from build123d import *

# Parameters (mm, degrees)
SKETCH_1_W      = 15
SKETCH_1_H      = 10
EXTRUDE_1_DEPTH = 5
FILLET_1_R      = 1.2


with BuildPart() as part:
    # 草图1 → 凸台-拉伸1 (new body)
    with BuildSketch(Plane(origin=(0, 0, 0), x_dir=(1, 0, 0), z_dir=(0, 1, 0))):
        Rectangle(SKETCH_1_W, SKETCH_1_H)
    extrude(amount=EXTRUDE_1_DEPTH)

    # 草图2 → 旋转1 (revolve)
    with BuildSketch(Plane.XY):
        with BuildLine():
            Line((-3.5, 6.5), (3.5, 6.5))
            ThreePointArc((3.5, 6.5), (4.560660172, 6.060660172), (5, 5))
            Line((5, 5), (-5, 5))
            ThreePointArc((-5, 5), (-4.560660172, 6.060660172), (-3.5, 6.5))
        make_face()
    revolve(axis=Axis((-7.5, 5, 0), (1, 0, 0)))

    # 圆角1
    fillet_1_edges = [part.edges().sort_by_distance(p)[0] for p in [
        (0, 5, 1.5),
        (4.560660172, 5, -1.060660172),
        (-4.560660172, 5, 1.060660172),
        (0, 5, -1.5),
    ]]
    fillet(fillet_1_edges, radius=FILLET_1_R)


solid = part.part
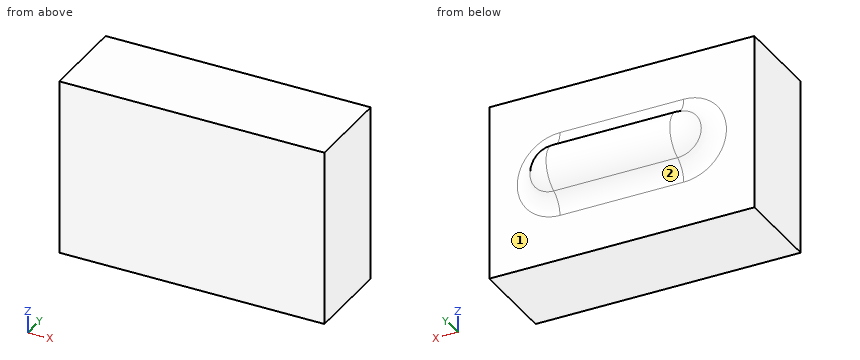
Check sheet for the modelled part. Datum: model origin and axes. Units: mm. Face numbers are marked on the shaded views. A direction names the side the tool comes from. Round coordinates to 2 decimals unless told otherwise and drop trailing zeros. Write each loop counter-clockwise with the first axis right and the second up, starting at its lowest first coordinate (ties: lowest second). Pieces come first, ordered by that corner, then holes. Notation, with made-up numbers: (72, 10) -> (88, 10) arc R18 cw to (88, 16) -> close; hole circle Ø8 at (74, 75). An arc over 180 degrees is marked (long way). Answer as CSV lines item,"result". Start each with the question number.
1) Section check C-C on x = 6.75. Enter the section's corners in (y, z).
2) Tool access check on the marked faces 1 and 2. Record the directions out of +Z, -Z, +X, -X, +Y, -Y that give a thin tool (end or side, any length) a straight path to the whole face; none if there is none.
3) Go/stop test with a flat-tipped pin: P1, Ø4, axis at x = 2.5, z = -4, coming from the +Y side. Record where the tip stops, or that it passes through.
4) Section check B-B on z = 3.5. Enter the section's corners in (x, y), and give its area (3 significant figures).
5) Section check A-A on x = 1.25. Enter the section's corners in (y, z).
6) Material ranges on line 1 (Y direction, x = -3, z = -2.5); line 2 (Z direction, x = -3.5, y = 6); line 3 (Y direction, x = 5.5, z = -0.25), recorded low to high. Write a range as from..to.
Found:
1,outline,"(0, -5) -> (5, -5) -> (5, 5) -> (0, 5) -> close"
2,face 1,"+Y"
2,face 2,"-Z, +X, -X, +Y"
3,P1,"stops at y = 5.08"
4,outline,"(-7.5, 0) -> (7.5, 0) -> (7.5, 5) -> (-7.5, 5) -> close"
4,area,"75.0 mm^2"
5,outline,"(0, -5) -> (5, -5) -> (5, -2.42) arc R1.2 cw to (5.67, -1.34) arc R1.5 ccw to (5.67, 1.34) arc R1.2 cw to (5, 2.42) -> (5, 5) -> (0, 5) -> close"
6,line 1,"y = 0..5"
6,line 2,"z = -1.12..1.12"
6,line 3,"y = 0..5.07"
